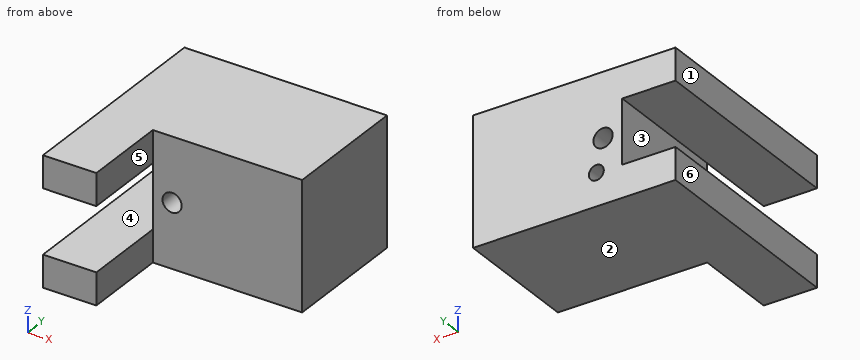
```python
from build123d import *

# Parameters (mm, degrees)
ESQUISSE1_W                = 70
ESQUISSE1_H                = 60
BOSS_EXTRU_1_DEPTH         = 60
ESQUISSE2_W                = 15
ESQUISSE2_H                = 60
BOSS_EXTRU_2_DEPTH         = 25
ESQUISSE3_W                = 25
ESQUISSE3_H                = 15
BOSS_EXTRU_3_DEPTH         = 40
TROU_TARAUD_M8X1_01_D      = 7
TROU_TARAUD_M8X1_01_DEPTH  = 21
TROU_TARAUD_M8X1_01_TIP    = 2.103012167
TROU_TARAUD_M10X1_02_D     = 9
TROU_TARAUD_M10X1_02_DEPTH = 25
TROU_TARAUD_M10X1_02_TIP   = 2.703872786
ENL_V_MAT_EXTRU_3_REACH    = 131.67
ESQUISSE4_R                = 4.5


with BuildPart() as part:
    # Esquisse1 → Boss.-Extru.1 (new body)
    with BuildSketch(Plane.XY):
        with Locations((-38.052617229, 47.387919463)):
            Rectangle(ESQUISSE1_W, ESQUISSE1_H)
    extrude(amount=BOSS_EXTRU_1_DEPTH)

    # Esquisse2 → Boss.-Extru.2 (add)
    with BuildSketch(Plane.ZY.offset(73.052617229)):
        with Locations((7.5, 47.387919463)):
            Rectangle(ESQUISSE2_W, ESQUISSE2_H)
        with Locations((52.5, 47.387919463)):
            Rectangle(ESQUISSE2_W, ESQUISSE2_H)
    extrude(amount=BOSS_EXTRU_2_DEPTH)

    # Esquisse3 → Boss.-Extru.3 (add)
    with BuildSketch(Plane.XZ.offset(-17.387919463)):
        with Locations((-85.552617229, 52.5)):
            Rectangle(ESQUISSE3_W, ESQUISSE3_H)
        with Locations((-85.552617229, 7.5)):
            Rectangle(ESQUISSE3_W, ESQUISSE3_H)
    extrude(amount=BOSS_EXTRU_3_DEPTH)

    # Trou taraudé M8x1.01
    with Locations(Plane(origin=(-60.909201033, 77.387919463, 15.33448507), x_dir=(0, 0, 1), z_dir=(0, 1, 0))):
        with Locations((0, 0)):
            Hole(TROU_TARAUD_M8X1_01_D / 2, depth=TROU_TARAUD_M8X1_01_DEPTH)
            with Locations((0, 0, -(TROU_TARAUD_M8X1_01_DEPTH + TROU_TARAUD_M8X1_01_TIP / 2))):  # 118° drill point
                Cone(0, TROU_TARAUD_M8X1_01_D / 2, TROU_TARAUD_M8X1_01_TIP, mode=Mode.SUBTRACT)

    # Trou taraudé M10x1.02
    with Locations(Plane(origin=(-64.052617229, 17.387919463, 30), x_dir=(0, 0, -1), z_dir=(0, -1, 0))):
        with Locations((0, 0)):
            Hole(TROU_TARAUD_M10X1_02_D / 2, depth=TROU_TARAUD_M10X1_02_DEPTH)
            with Locations((0, 0, -(TROU_TARAUD_M10X1_02_DEPTH + TROU_TARAUD_M10X1_02_TIP / 2))):  # 118° drill point
                Cone(0, TROU_TARAUD_M10X1_02_D / 2, TROU_TARAUD_M10X1_02_TIP, mode=Mode.SUBTRACT)

    # Esquisse4 → Enlèv. mat.-Extru.3 (cut, up to next)
    with BuildSketch(Plane.XZ.offset(-17.387919463), mode=Mode.PRIVATE) as enl_v_mat_extru_3_sk1:
        with Locations(Location((-64.052617229, 30, 0), (0, 0, 270))):
            Circle(ESQUISSE4_R)
    enl_v_mat_extru_3_tool1 = extrude(enl_v_mat_extru_3_sk1.sketch, amount=-ENL_V_MAT_EXTRU_3_REACH, mode=Mode.PRIVATE) & part.part
    add(enl_v_mat_extru_3_tool1.solids().sort_by_distance((-64.052617, 17.387919, 30))[0], mode=Mode.SUBTRACT)


solid = part.part
```
The model under review builds one solid part; all positions refer to its coordinate system, in mm. Face numbers are marked on the shaded views. A direction names the side the tool comes from. Give positions to 0.01 mm unless a question says otherwise; leave off trailing zeros. Write each loop counter-clockwise with the first axis right and the second up, starting at its lowest first coordinate (ties: lowest second). Pieces come first, ordered by that corner, then holes. Notation, with made-up numbers: M -35,73.25 L -22,73.25 A30 cw -22,104.25 Z; hole C 44,-8.75 d9. An arc over 180 degrees is marked long. Answer in a Markdown table with one row per item.
Item 1: Draft analysis for pull direction Z (two halves, no side actions). For the marked faces 1, 2 and 3, state which applies: +Z half, -Z half, draft (parallel to the pull), parting line (faces both ways), or undercut.
Check sheet entries:
| item | result |
|---|---|
| face 1 | draft |
| face 2 | -Z half |
| face 3 | undercut |
Item 2: Add section D-D on y = 67.5. Give the boundary of the cut face in (x, z), plus the area to 3 significant figures.
Check sheet entries:
| item | result |
|---|---|
| outline | M -98.05,0 L -3.05,0 L -3.05,60 L -98.05,60 L -98.05,45 L -73.05,45 L -73.05,15 L -98.05,15 Z; hole C -64.05,30 d9; hole C -60.91,15.33 d7 |
| area | 4,850 mm2 |
Item 3: Add section A-A on y = -17. Give the boundary of the cut face in (x, z).
Check sheet entries:
| item | result |
|---|---|
| outline | M -98.05,0 L -73.05,0 L -73.05,15 L -98.05,15 Z; M -98.05,45 L -73.05,45 L -73.05,60 L -98.05,60 Z |
Item 4: Add section B-B on x = -78. Give the boundary of the cut face in (y, z).
Check sheet entries:
| item | result |
|---|---|
| outline | M -22.61,0 L 77.39,0 L 77.39,15 L -22.61,15 Z; M -22.61,45 L 77.39,45 L 77.39,60 L -22.61,60 Z |
Item 5: For P1, Ø7.5, axis at x = -84, y = 16, coming from the -Z side; P2, Ø12, axis at x = -63, y = -8, coming from the -Z side; P3, Ø1, axis at y = 5.5, z = 9.5, coming from the +X side; P4, Ø9, axis at y = 61.5, z = 35, coming from the -X side, all flat-tipped, find the tip position at first contact; note any pin that passes through.
Check sheet entries:
| item | result |
|---|---|
| P1 | z = 0 |
| P2 | through |
| P3 | x = -73.05 |
| P4 | x = -73.05 |
Item 6: Add section C-C on z = 48. Give the boundary of the cut face in (x, y), plus the area to 3 significant figures.
Check sheet entries:
| item | result |
|---|---|
| outline | M -98.05,-22.61 L -73.05,-22.61 L -73.05,17.39 L -3.05,17.39 L -3.05,77.39 L -98.05,77.39 Z |
| area | 6,700 mm2 |
Item 7: For line 1 along Z through (x, y) = (-85.5, 23.5); line 2 along X through (y, z) = (43.5, 30); line 3 along X through (y, z) = (-3.5, 51.5), list the stretches that pass through material, from the lowest coordinate up.
Check sheet entries:
| item | result |
|---|---|
| line 1 | 0 to 15, 45 to 60 |
| line 2 | -73.05 to -68.55, -59.55 to -3.05 |
| line 3 | -98.05 to -73.05 |
Item 8: Tool access review of the marked faces 4, 5 and 6: name each direction out of +Z, -Z, +X, -X, +Y, -Y from which nothing blocks a thin tool from reaching the whole face with its end or side.
Check sheet entries:
| item | result |
|---|---|
| face 4 | -X, +Y, -Y |
| face 5 | +Z, -Z, +X, -Y |
| face 6 | +Z, -Z, -X, +Y, -Y |
